Could you check a few things on this model? Use its own coordinates, in mm. A direction names the side the tool comes from. Coordinates: 2 decimals unless noted, no trailing zeros. Order: outer loops, then holes, each group sorted by start corner. A loop starts at its lowest first (then second) coordinate and runs counter-clockwise, first axis right, second up. Notation, with made-up numbers: M -11,-3 L 45,-3 A16 cw 45,14 Z; hole C -21,-27.5 d11. An arc over 180 degrees is marked long. One line per question, with ' | ' between items. Start each with the question number.
from build123d import *

# Parameters (mm, degrees)
BOSS_EXTRUDE1_DEPTH = 10
SKETCH3_R           = 3.5
CUT_EXTRUDE1_DEPTH  = 4
SKETCH4_R           = 1.55
CUT_EXTRUDE2_DEPTH  = 22


with BuildPart() as part:
    # Sketch1 → Boss-Extrude1 (new body)
    with BuildSketch(Plane.XY):
        with BuildLine():
            Line((-10, 0), (-10, 30))
            ThreePointArc((-10, 30), (0, 40), (10, 30))
            Line((10, 30), (10, 0))
            ThreePointArc((10, 0), (0, -10), (-10, 0))
        make_face()
    extrude(amount=BOSS_EXTRUDE1_DEPTH)

    # Sketch3 → Cut-Extrude1 (cut)
    with BuildSketch(Plane.XY.offset(10)):
        Circle(SKETCH3_R)
        with Locations(Location((0, 30, 0), (0, 0, 180))):
            Circle(SKETCH3_R)
    extrude(amount=-CUT_EXTRUDE1_DEPTH, mode=Mode.SUBTRACT)

    # Sketch4 → Cut-Extrude2 (cut)
    with BuildSketch(Plane.XY.offset(6)):
        Circle(SKETCH4_R)
        with Locations((0, 30)):
            Circle(SKETCH4_R)
    extrude(amount=-CUT_EXTRUDE2_DEPTH, mode=Mode.SUBTRACT)


solid = part.part
(1) We'd pull the mould along X, two halves only. Please class faces 1 (the flat face through (10, 15, 5)), 2 (the cylindrical face through (0, -10, 5)), 3 (the cylindrical face through (-0.202, 31.537, 3.042)): +X half, -X half, draft (parallel to the pull), parting line (faces both ways), or undercut.
(2) Imagine slicing it at B-B, the plane z = 8. Write out the boundary of the cut face in (x, y), plus the area to 3 significant figures.
(3) If I drill on line 1 along Y through (x, z) = (0, 7.35); line 2 along Y through (x, z) = (0, 1.7); line 3 along Z through (x, y) = (-1.5, 33), over which ranges is the centre line in solid material (lowest first)? Write a range as from..to.
(4) Imagine slicing it at D-D, the plane z = 3.5. Write out the boundary of the cut face in (x, y).
(5) Imagine slicing it at A-A, the plane x = 0. Write out the boundary of the cut face in (y, z).
(6) Imagine slicing it at C-C, the plane y = -3. Write out the boundary of the cut face in (x, z), plus the area to 3 significant figures.
(7) On a 3-axis mill with a long thin cutter (end or side, diameter ignored), from which of +Z, -Z, +X, -X, +Y, -Y can I reach the whole of each face in a straight line? I mean faces 4 (the cylindrical face through (0, 40, 5)), 5 (the flat face through (1, -2, 6)). Say none if no direction works.
(8) For P1, Ø5, axis at x = 6, z = 2, coming from the +Y side; P2, Ø3, axis at x = -6.5, z = 4, coming from the +Y side; P3, Ø4, axis at x = 0, y = 30, coming from the +Z side, each with a flat end and sliding along its axis, tell me the tip position at first contact or that it passes through.
Answers:
1) face 1: +X half | face 2: parting line | face 3: undercut
2) outline: M -10,0 A10 ccw 10,0 L 10,30 A10 ccw -10,30 Z; hole C 0,0 d7; hole C 0,30 d7 | area: 837 mm²
3) line 1: -10..-3.5, 3.5..26.5, 33.5..40 | line 2: -10..-1.55, 1.55..28.45, 31.55..40 | line 3: 0..6
4) outline: M -10,0 A10 ccw 10,0 L 10,30 A10 ccw -10,30 Z; hole C 0,0 d3.1; hole C 0,30 d3.1
5) outline: M -10,0 L -1.55,0 L -1.55,6 L -3.5,6 L -3.5,10 L -10,10 Z; M 1.55,0 L 28.45,0 L 28.45,6 L 26.5,6 L 26.5,10 L 3.5,10 L 3.5,6 L 1.55,6 Z; M 31.55,0 L 40,0 L 40,10 L 33.5,10 L 33.5,6 L 31.55,6 Z
6) outline: M -9.54,0 L 9.54,0 L 9.54,10 L 1.8,10 L 1.8,6 L -1.8,6 L -1.8,10 L -9.54,10 Z | area: 176 mm²
7) face 4: +Z, -Z, +Y | face 5: +Z
8) P1: y = 39.37 | P2: y = 38.66 | P3: z = 6
